Design review of the part built by this model. Coordinates are the model's own, in mm. Face numbers are marked on the shaded views. A direction names the side the tool comes from. Coordinates: 2 decimals unless noted, no trailing zeros. Write each loop counter-clockwise with the first axis right and the second up, starting at its lowest first coordinate (ties: lowest second). Pieces come first, ordered by that corner, then holes. Notation, with made-up numbers: (6, -8) - (54, -8) arc R15 cw to (54, 9) - close; hole circle Ø1 at (70.25, 7.5). An arc over 180 degrees is marked (long way). Answer as CSV lines item,"result". Start each with the question number.
Q1. We need section C-C (z = -3). Write out the cut boundary in (x, y), plus the area to 3 significant figures.
Q2. We need section B-B (y = 32.5). Write out the cut boundary in (x, z).
Q3. Machinability: for the marked faces 1 and 2, which of the approach directions +Z, -Z, +X, -X, +Y, -Y give a long, thin tool a straight path to every point of the face, cutting with its end or side? Answer none if there is none.
Q4. We need section D-D (x = 10.5). Write out the cut boundary in (y, z), plus the area to 3 significant figures.
Q5. We need section A-A (x = 0). Write out the cut boundary in (y, z).
Q6. For line 1 along Z through (x, y) = (6, -29.5); line 2 along Y through (x, z) = (12.5, 5); line 3 along X through (y, z) = (-17, 3), list the stretches that pass through material, from the lowest coordinate up. Write a range as [from, to].
Q7. Clearance check with flat-ended pins moving along their axes: pin 1 (3 mm diameter, centred on x = -20.5, z = -1, fed in from -Y); pin 2 (22.5 mm diameter, centred on x = -10.5, y = -7.5, fed in from -Z). State where each tip first meets the part, or that it passes through.
from build123d import *

# Parameters (mm, degrees)
F0_W     = 90.572778
F0_H     = 85.716326
F1_DEPTH = 25.4
F2_R     = 5.08
F3_R     = 11.744353
F4_DEPTH = 25.4


with BuildPart() as f1:
    # F0 (on Top) → F1 (new body)
    with BuildSketch(Plane.XY):
        with Locations((1.0927, 8.741608)):
            Rectangle(F0_W, F0_H)
    extrude(amount=F1_DEPTH)

    # F2
    f2_edges = [f1.edges().sort_by_distance(p)[0] for p in [
        (46.379089, 51.599771, 12.7),
        (-44.193689, 51.599771, 12.7),
        (1.0927, 51.599771, 0),
        (1.0927, 51.599771, 25.4),
        (46.379089, -34.116555, 12.7),
        (46.379089, 8.741608, 0),
        (46.379089, 8.741608, 25.4),
        (-44.193689, -34.116555, 12.7),
        (-44.193689, 8.741608, 0),
        (-44.193689, 8.741608, 25.4),
        (1.0927, -34.116555, 0),
        (1.0927, -34.116555, 25.4),
    ]]
    fillet(f2_edges, radius=F2_R)

    # F3 (on face) → F4 (join)
    with BuildSketch(Plane(origin=(0, 0, 0), x_dir=(1, 0, 0), z_dir=(0, 0, -1))):
        with Locations((0, -14.89311)):
            Circle(F3_R)
    extrude(amount=F4_DEPTH)


solid = f1.part
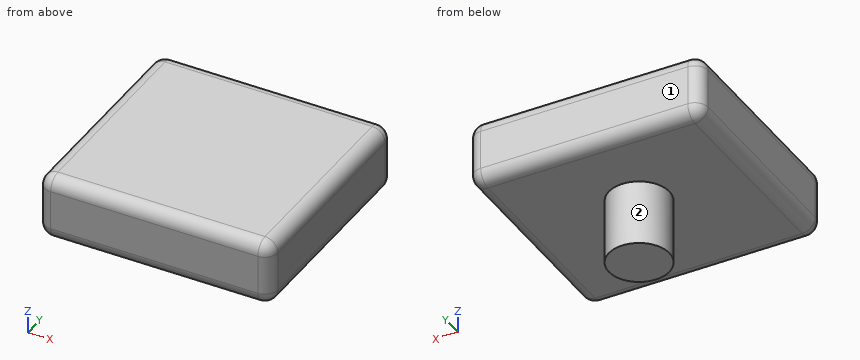
Results list:
1,outline,"circle Ø23.49 at (0, 14.89)"
1,area,"433 mm2"
2,outline,"(-44.19, 5.08) arc R5.08 ccw to (-39.11, 0) - (41.3, 0) arc R5.08 ccw to (46.38, 5.08) - (46.38, 20.32) arc R5.08 ccw to (41.3, 25.4) - (-39.11, 25.4) arc R5.08 ccw to (-44.19, 20.32) - close"
3,face 1,"+Z, -Z, +X, -X, +Y"
3,face 2,"-Z"
4,outline,"(-34.12, 5.08) arc R5.08 ccw to (-29.04, 0) - (9.63, 0) - (9.63, -25.4) - (20.15, -25.4) - (20.15, 0) - (46.52, 0) arc R5.08 ccw to (51.6, 5.08) - (51.6, 20.32) arc R5.08 ccw to (46.52, 25.4) - (-29.04, 25.4) arc R5.08 ccw to (-34.12, 20.32) - close"
4,area,"2,420 mm2"
5,outline,"(-34.12, 5.08) arc R5.08 ccw to (-29.04, 0) - (3.15, 0) - (3.15, -25.4) - (26.64, -25.4) - (26.64, 0) - (46.52, 0) arc R5.08 ccw to (51.6, 5.08) - (51.6, 20.32) arc R5.08 ccw to (46.52, 25.4) - (-29.04, 25.4) arc R5.08 ccw to (-34.12, 20.32) - close"
6,line 1,"z = [0.02, 25.38]"
6,line 2,"y = [-34.12, 51.6]"
6,line 3,"x = [-43.75, 45.93]"
7,pin 1,"stops at y = -31.23"
7,pin 2,"stops at z = 0"
